Could you check a few things on this model? Use its own coordinates, in mm. Face numbers are marked on the shaded views. A direction names the side the tool comes from. Give positions to 0.01 mm unless a question says otherwise; leave off trailing zeros. Write each loop counter-clockwise with the first axis right and the second up, starting at its lowest first coordinate (ties: lowest second). Pieces come first, ordered by that corner, then holes. Notation, with made-up numbers: (66, -20) -> (71, -20) arc R23 cw to (71, 5) -> close; hole circle Ø4 at (60, -18). An arc over 180 degrees is marked (long way). Write item = value, one per line. Start each with the question number.
```python
from build123d import *

# Parameters (mm, degrees)
EXTRUDE_1_DEPTH     = 2.5
BOSS_EXTRUDE3_START = -2.5
BOSS_EXTRUDE3_DEPTH = 5


with BuildPart() as part:
    # Эскиз1 → Бобышка-Вытянуть1 (new, symmetric)
    with BuildSketch(Plane.XY):
        with BuildLine():
            Line((3.269215058, 15.662446581), (2.569872981, 14.451150572))
            Line((2.569872981, 14.451150572), (11.230127019, 9.451150572))
            Line((11.230127019, 9.451150572), (11.929469096, 10.662446581))
            ThreePointArc((11.929469096, 10.662446581), (15.454813221, -4.141104722), (5, -15.198684154))
            Line((5, -15.198684154), (5, -13.8))
            Line((5, -13.8), (0, -13.8))
            Line((0, -13.8), (-5, -13.8))
            Line((-5, -13.8), (-5, -15.198684154))
            ThreePointArc((-5, -15.198684154), (-15.454813221, -4.141104722), (-11.929469096, 10.662446581))
            Line((-11.929469096, 10.662446581), (-11.230127019, 9.451150572))
            Line((-11.230127019, 9.451150572), (-2.569872981, 14.451150572))
            Line((-2.569872981, 14.451150572), (-3.269215058, 15.662446581))
            ThreePointArc((-3.269215058, 15.662446581), (0, 16), (3.269215058, 15.662446581))
        make_face()
        with BuildLine():
            Line((-2.5, -2.359609465), (-2.5, -3.304777846))
            ThreePointArc((-2.5, -3.304777846), (0, -12.85), (2.5, -3.304777846))
            Line((2.5, -3.304777846), (2.5, -2.359609465))
            ThreePointArc((2.5, -2.359609465), (4.180016715, -1.604605606), (5.649137352, -0.493672869))
            Line((5.649137352, -0.493672869), (6.41139529, -0.943209602))
            ThreePointArc((6.41139529, -0.943209602), (12.678644072, -2.027149068), (8.69732788, 2.932936963))
            Line((8.69732788, 2.932936963), (7.935069942, 3.382473696))
            ThreePointArc((7.935069942, 3.382473696), (0, 13.65), (-7.935069942, 3.382473696))
            Line((-7.935069942, 3.382473696), (-8.69732788, 2.932936963))
            ThreePointArc((-8.69732788, 2.932936963), (-12.678644072, -2.027149068), (-6.41139529, -0.943209602))
            Line((-6.41139529, -0.943209602), (-5.649137352, -0.493672869))
            ThreePointArc((-5.649137352, -0.493672869), (-4.180016715, -1.604605606), (-2.5, -2.359609465))
        make_face(mode=Mode.SUBTRACT)
    extrude(amount=EXTRUDE_1_DEPTH, both=True)

    # Sketch2 → Boss-Extrude3 (add)
    with BuildSketch(Plane.XY.offset(BOSS_EXTRUDE3_START)):
        with BuildLine():
            ThreePointArc((-5, -15.198684154), (-14.947767484, -5.706509199), (-13.856406461, 8))
            Line((-13.856406461, 8), (-14.722431864, 8.5))
            ThreePointArc((-14.722431864, 8.5), (-15.822781238, -6.216075442), (-5, -16.248076809))
            Line((-5, -16.248076809), (-5, -15.198684154))
        make_face()
        with BuildLine():
            Line((14.722431864, 8.5), (13.856406461, 8))
            ThreePointArc((13.856406461, 8), (14.947767484, -5.706509199), (5, -15.198684154))
            Line((5, -15.198684154), (5, -16.248076809))
            ThreePointArc((5, -16.248076809), (15.822781238, -6.216075442), (14.722431864, 8.5))
        make_face()
    extrude(amount=BOSS_EXTRUDE3_DEPTH)


solid = part.part
```
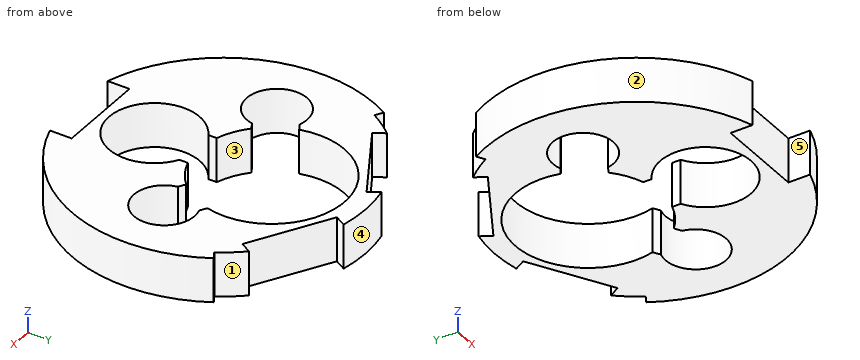
(1) We'd pull the mould along Y, two halves only. Please class the marked faces 1, 2 and 3: released by +Y, released by -Y, zero draft, split by the parting line, or undercut.
(2) On a 3-axis mill with a long thin cutter (end or side, diameter ignored), from which of +Z, -Z, +X, -X, +Y, -Y can I reach the whole of each face in a straight line? I mean the marked faces 4 and 5. Say none if no direction works.
(3) Imagine slicing it at A-A (x = 0). Please give me the cut outline in (y, z).
(4) If I drill on line 1 along X through (y, z) = (-0.3, -0.4); line 2 along Y through (x, z) = (-4, 1.1); line 3 along X through (y, z) = (-2.5, 1.5), over which ranges is the centre line in solid material (lowest first)? Write a range as from..to.
(5) Imagine slicing it at C-C (z = -0.95). Please give me the cut outline in (x, y), then the cut area to 3 significant figures.
(6) Imagine slicing it at D-D (x = 4). Please give me the cut outline in (y, z).
(7) I'm going to push flat-ended pins straight in: pin 1 (1 mm diameter, centred on x = 2, z = -0.5, fed in from -Y); pin 2 (2.5 mm diameter, centred on y = -15, z = -0.5, fed in from +X); pin 3 (2 mm diameter, centred on y = -14.5, z = -1, fed in from -X). Where does each tip first touch, or does it pass through?
(8) Imagine slicing it at B-B (y = 5.45). Please give me the cut outline in (x, z).
Answers below:
q1.face_1 = released by +Y
q1.face_2 = split by the parting line
q1.face_3 = undercut
q2.face_4 = +Z, -Z, +Y
q2.face_5 = +Z, -Z, -Y
q3.outline = (-13.8, -2.5) -> (-12.85, -2.5) -> (-12.85, 2.5) -> (-13.8, 2.5) -> close; (13.65, -2.5) -> (16, -2.5) -> (16, 2.5) -> (13.65, 2.5) -> close
q4.line_1 = -17..-13.15, 13.15..17
q4.line_2 = -13.8..-10.91, -4.59..-1.71, 12.61..13.63
q4.line_3 = -16.82..-12.34, -7.16..-2.5, 2.5..7.16, 12.34..16.82
q5.outline = (-14.72, 8.5) arc R17 ccw to (-5, -16.25) -> (-5, -13.8) -> (5, -13.8) -> (5, -16.25) arc R17 ccw to (14.72, 8.5) -> (13.86, 8) arc R16 ccw to (11.93, 10.66) -> (11.23, 9.45) -> (2.57, 14.45) -> (3.27, 15.66) arc R16 ccw to (-3.27, 15.66) -> (-2.57, 14.45) -> (-11.23, 9.45) -> (-11.93, 10.66) arc R16 ccw to (-13.86, 8) -> close; hole (-8.7, 2.93) arc R3.4 ccw (long way) to (-6.41, -0.94) -> (-5.65, -0.49) arc R8.2 ccw to (-2.5, -2.36) -> (-2.5, -3.3) arc R5.1 ccw (long way) to (2.5, -3.3) -> (2.5, -2.36) arc R8.2 ccw to (5.65, -0.49) -> (6.41, -0.94) arc R3.4 ccw (long way) to (8.7, 2.93) -> (7.94, 3.38) arc R8.2 ccw (long way) to (-7.94, 3.38) -> close
q5.area = 438 mm^2
q6.outline = (-13.8, -2.5) -> (-10.91, -2.5) -> (-10.91, 2.5) -> (-13.8, 2.5) -> close; (-4.59, -2.5) -> (-1.71, -2.5) -> (-1.71, 2.5) -> (-4.59, 2.5) -> close; (12.61, -2.5) -> (13.63, -2.5) -> (13.63, 2.5) -> (12.61, 2.5) -> close
q7.pin_1 = -13.8
q7.pin_2 = 10
q7.pin_3 = -10.33
q8.outline = (-16.1, -2.5) -> (-8.2, -2.5) -> (-8.2, 2.5) -> (-16.1, 2.5) -> close; (8.2, -2.5) -> (16.1, -2.5) -> (16.1, 2.5) -> (8.2, 2.5) -> close
